Can you work these out from the model? Positions are in its coordinate system, mm. Round coordinates to 2 decimals unless told otherwise and drop trailing zeros. Loops run counter-clockwise (first coordinate to the right, second up) from the corner with the lowest first, then second, coordinate; pieces in that order, holes last.
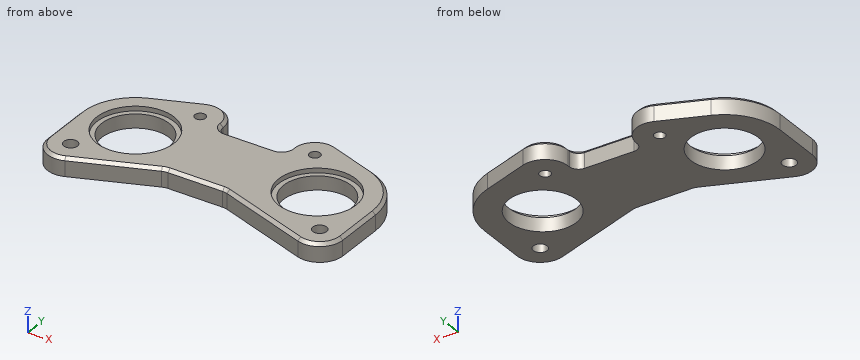
```python
from build123d import *

# Parameters (mm, degrees)
F0_R     = 4.5
F0_R_2   = 22
F0_R_3   = 3.5
F1_DEPTH = 12
F2_R     = 25.2
F3_DEPTH = 3
F4_SIZE  = 2


# Not quite as in the source:
# - ends of sketch curves that miss each other by under 0.0002 mm in the source are joined


with BuildPart() as f1:
    # F0 (on Top) → F1 (new body)
    with BuildSketch(Plane.XY):
        with BuildLine():
            Line((-96.25, -7.835472), (-96.25, -39.300472))
            ThreePointArc((-96.25, -39.300472), (-89.6603385796, -51.720866719), (-75.6811726698, -53.2284353172))
            Line((-75.6811726698, -53.2284353172), (-25.901923657, -33.3251628629))
            ThreePointArc((-25.901923657, -33.3251628629), (-24.0797305928, -32.7907701516), (-22.189372, -32.610472))
            Line((-22.189372, -32.610472), (13.41096, -32.610472))
            ThreePointArc((13.41096, -32.610472), (15.0445629213, -32.7448072228), (16.6342757601, -33.1442037009))
            Line((16.6342757601, -33.1442037009), (76.4150264593, -53.4998741564))
            ThreePointArc((76.4150264593, -53.4998741564), (89.9814201421, -51.4972872524), (96.25, -39.300472))
            Line((96.25, -39.300472), (96.25, -7.385472))
            ThreePointArc((96.25, -7.385472), (89.1771507076, 14.6451910108), (70.602136617, 28.4417181588))
            Line((70.602136617, 28.4417181588), (40.3905414757, 38.7289301785))
            ThreePointArc((40.3905414757, 38.7289301785), (26.82414783, 36.7263432324), (20.555568, 24.529528))
            Line((20.555568, 24.529528), (20.555568, 23.389528))
            ThreePointArc((20.555568, 23.389528), (18.7982086871, 19.1468873129), (14.555568, 17.389528))
            Line((14.555568, 17.389528), (-17.637618, 17.389528))
            ThreePointArc((-17.637618, 17.389528), (-21.8802586871, 19.1468873129), (-23.637618, 23.389528))
            Line((-23.637618, 23.389528), (-23.637618, 23.629528))
            ThreePointArc((-23.637618, 23.629528), (-30.2272793638, 36.0499226807), (-44.2064452032, 37.557491368))
            Line((-44.2064452032, 37.557491368), (-73.4226694122, 25.875948235))
            ThreePointArc((-73.4226694122, 25.875948235), (-90.0062904382, 12.5210187268), (-96.25, -7.835472))
        make_face()
        with Locations((-81.25, -39.300472)):
            Circle(F0_R, mode=Mode.SUBTRACT)
        with Locations((-59.943809, -7.835472)):
            Circle(F0_R_2, mode=Mode.SUBTRACT)
        with Locations((81.25, -39.300472)):
            Circle(F0_R, mode=Mode.SUBTRACT)
        with Locations((-38.637618, 23.629528)):
            Circle(F0_R_3, mode=Mode.SUBTRACT)
        with Locations((58.402784, -7.385472)):
            Circle(F0_R_2, mode=Mode.SUBTRACT)
        with Locations((35.555568, 24.529528)):
            Circle(F0_R_3, mode=Mode.SUBTRACT)
    extrude(amount=F1_DEPTH)

    # F2 (on face) → F3 (cut)
    with BuildSketch(Plane.XY.offset(12)):
        with Locations((-59.943809, -7.835472)):
            Circle(F2_R)
        with Locations((58.402784, -7.385472)):
            Circle(F2_R)
    extrude(amount=-F3_DEPTH, mode=Mode.SUBTRACT)

    # F4
    f4_edges = [f1.edges().sort_by_distance(p)[0] for p in [
        (-58.814557, 31.71672, 12),
    ]]
    chamfer(f4_edges, length=F4_SIZE)


solid = f1.part
```
(1) For pin 1 (1.5 mm diameter, centred on x = 41, z = 5.5, fed in from -Y); pin 2 (1.5 mm diameter, centred on x = -26, z = 7, fed in from -Y); pin 3 (3 mm diameter, centred on x = -6, z = 6, fed in from +Y), each with a flat end and sliding along its axis, tell me the tip position at first contact or that it passes through.
(2) Suppose I cut it at C-C (y = 6). Give the number of separate pieces and of enclosed holes in the cut face, then the cut area to 3 significant figures.
(3) Suppose I cut it at A-A (z = 4.5). Write out the boundary of the cut face in (x, y), then the cut area to 3 significant figures.
(4) If I drill on line 1 (X direction, y = -27.5, z = 11.5); line 2 (X direction, y = -5.5, z = 10); line 3 (Y direction, x = -65, z = 1.25), over which ranges is the centre line in solid material (lowest first)?
(5) Suppose I cut it at B-B (x = -50.5). Write out the boundary of the cut face in (y, z).
(6) Suppose I cut it at D-D (x = 44.5). Write out the boundary of the cut face in (y, z).
Check result:
1. pin 1: stops at y = -41.7
1. pin 2: stops at y = -33.66
1. pin 3: stops at y = 17.39
2. separate pieces: 3
2. enclosed holes: 0
2. area: 1,370 mm2
3. outline: (-96.25, -39.3) arc R15 ccw to (-75.68, -53.23) - (-25.9, -33.33) arc R10 cw to (-22.19, -32.61) - (13.41, -32.61) arc R10 cw to (16.63, -33.14) - (76.42, -53.5) arc R15 ccw to (96.25, -39.3) - (96.25, -7.39) arc R37.85 ccw to (70.6, 28.44) - (40.39, 38.73) arc R15 ccw to (20.56, 24.53) - (20.56, 23.39) arc R6 cw to (14.56, 17.39) - (-17.64, 17.39) arc R6 cw to (-23.64, 23.39) - (-23.64, 23.63) arc R15 ccw to (-44.21, 37.56) - (-73.42, 25.88) arc R36.31 ccw to (-96.25, -7.84) - close; hole circle Ø9 at (-81.25, -39.3); hole circle Ø44 at (-59.94, -7.84); hole circle Ø7 at (-38.64, 23.63); hole circle Ø7 at (35.56, 24.53); hole circle Ø44 at (58.4, -7.39); hole circle Ø9 at (81.25, -39.3)
3. area: 10,000 mm2
4. line 1: x = -94.75 to -75.7, -44.18 to 43.22, 73.58 to 94.75
4. line 2: x = -96.17 to -85.04, -34.85 to 33.27, 83.53 to 96.2
4. line 3: y = -48.96 to -29.25, 13.58 to 29.24
5. outline: (-43.16, 0) - (-27.71, 0) - (-27.71, 9) - (-31.2, 9) - (-31.2, 12) - (-41.01, 12) - (-43.16, 10) - close; (12.03, 0) - (35.04, 0) - (35.04, 10) - (32.89, 12) - (15.53, 12) - (15.53, 9) - (12.03, 9) - close
6. outline: (-42.63, 0) - (-24.44, 0) - (-24.44, 9) - (-28.4, 9) - (-28.4, 12) - (-40.52, 12) - (-42.63, 10) - close; (9.66, 0) - (37.33, 0) - (37.33, 10) - (35.22, 12) - (13.63, 12) - (13.63, 9) - (9.66, 9) - close
